Read the model definition and answer for the solid it produces. Units are mm, in the model's axes. Round coordinates to 2 decimals unless told otherwise and drop trailing zeros. Write each loop counter-clockwise with the first axis right and the second up, starting at its lowest first coordinate (ties: lowest second). Pieces come first, ordered by that corner, then holes. Notation, with made-up numbers: (-11.5, -27.75) -> (6.5, -27.75) arc R12 ccw to (6.5, -16.75) -> close; hole circle Ø8 at (67, 83). An arc over 180 degrees is marked (long way). Return JSON: item names as keys, results as strings.
from build123d import *

# Parameters (mm, degrees)
F0_R     = 2.25
F0_W     = 6
F0_H     = 2
F0_R_2   = 3
F1_DEPTH = 5


with BuildPart() as f1:
    # F0 (on Top) → F1 (new body)
    with BuildSketch(Plane.XY):
        with BuildLine():
            ThreePointArc((-170, -8), (-169.414214, -9.414214), (-168, -10))
            Line((-168, -10), (468, -10))
            ThreePointArc((468, -10), (469.414214, -9.414214), (470, -8))
            Line((470, -8), (470, 70))
            Line((470, 70), (449.5, 70))
            Line((449.5, 70), (449.5, 90))
            Line((449.5, 90), (210, 90))
            Line((210, 90), (210, 70))
            Line((210, 70), (90, 70))
            Line((90, 70), (90, 90))
            Line((90, 90), (-149.5, 90))
            Line((-149.5, 90), (-149.5, 70))
            Line((-149.5, 70), (-170, 70))
            Line((-170, 70), (-170, -8))
        make_face()
        with Locations((-160, -5)):
            Circle(F0_R, mode=Mode.SUBTRACT)
        with Locations((-60, -4)):
            Rectangle(F0_W, F0_H, mode=Mode.SUBTRACT)
        with Locations((-70, 0)):
            Circle(F0_R_2, mode=Mode.SUBTRACT)
        with Locations((-60, 4)):
            Rectangle(F0_W, F0_H, mode=Mode.SUBTRACT)
        with Locations((80, -4)):
            Rectangle(F0_W, F0_H, mode=Mode.SUBTRACT)
        with Locations((70, 0)):
            Circle(F0_R_2, mode=Mode.SUBTRACT)
        with Locations((80, 4)):
            Rectangle(F0_W, F0_H, mode=Mode.SUBTRACT)
        with Locations((220, -4)):
            Rectangle(F0_W, F0_H, mode=Mode.SUBTRACT)
        with Locations((230, 0)):
            Circle(F0_R_2, mode=Mode.SUBTRACT)
        with Locations((220, 4)):
            Rectangle(F0_W, F0_H, mode=Mode.SUBTRACT)
        with Locations((360, -4)):
            Rectangle(F0_W, F0_H, mode=Mode.SUBTRACT)
        with Locations((370, 0)):
            Circle(F0_R_2, mode=Mode.SUBTRACT)
        with Locations((460, -5)):
            Circle(F0_R, mode=Mode.SUBTRACT)
        with Locations((360, 4)):
            Rectangle(F0_W, F0_H, mode=Mode.SUBTRACT)
        with Locations((80, 80)):
            Circle(F0_R, mode=Mode.SUBTRACT)
    extrude(amount=F1_DEPTH)


solid = f1.part
Item 1: Flat-ended cylindrical pins translate along their axes: pin 1 (2 mm diameter, centred on y = 78, z = 4.5, fed in from +X); pin 2 (1.5 mm diameter, centred on y = 75.5, z = 2, fed in from -X). Find the tip coordinate at first contact, or state that the pin passes through.
Worked answers:
{"pin 1": "stops at x = 449.5", "pin 2": "stops at x = -149.5"}
Item 2: Section A-A (x = 120) is taken. Give the vertices of the cut face in (y, z), then the cut area to 3 significant figures.
Worked answers:
{"outline": "(-10, 0) -> (70, 0) -> (70, 5) -> (-10, 5) -> close", "area": "400 mm2"}
Item 3: Section B-B (z = 0.9) is taken. State how many separate pieces and enclosed holes the cut face has, then the cut area to 3 significant figures.
Worked answers:
{"separate pieces": "1", "enclosed holes": "15", "area": "60,500 mm2"}
Item 4: Straight lines are drawn through the part: L1, parallel to Y at x = 222.5, z = 3.1; L2, parallel to X at y = -0.5, z = 0.8; L3, parallel to X at y = 83, z = 0.4. For each, find the intervals that lie inside material, in ascending order. Write a range as [from, to].
Worked answers:
{"L1": "y = [-10, -5], [-3, 3], [5, 90]", "L2": "x = [-170, -72.96], [-67.04, 67.04], [72.96, 227.04], [232.96, 367.04], [372.96, 470]", "L3": "x = [-149.5, 90], [210, 449.5]"}
